Can you work these out from the model? Positions are in its coordinate system, mm. A direction names the side the tool comes from. Give positions to 0.01 mm unless a question says otherwise; leave off trailing zeros. Loops run counter-clockwise (first coordinate to the right, second up) from the corner with the lowest first, then second, coordinate; pieces in that order, holes last. Notation, with made-up numbers: M 20,7 L 45,7 A8 ccw 45,22 Z; hole C -23.5,70 d7. An arc over 180 degrees is marked long. Use CSV: the item, a comma, the result in double quotes.
from build123d import *

# Parameters (mm, degrees)
BOSS_EXTRUDE3_DEPTH  = 2.5
BOSS_EXTRUDE4_DEPTH  = 2.5
BOSS_EXTRUDE5_DEPTH  = 10.5
BOSS_EXTRUDE8_DEPTH  = 11
BOSS_EXTRUDE9_DEPTH  = 11
SKETCH8_W            = 84
SKETCH8_H            = 2
BOSS_EXTRUDE11_DEPTH = 4
SKETCH9_W            = 6
SKETCH9_H            = 7.053661792
CUT_EXTRUDE1_DEPTH   = 28
SKETCH10_W           = 6
SKETCH10_H           = 6.438726715
CUT_EXTRUDE4_DEPTH   = 11
SKETCH11_R           = 1.5
CUT_EXTRUDE5_DEPTH   = 14
SKETCH13_R           = 1.5
CUT_EXTRUDE6_DEPTH   = 14
SKETCH15_R           = 1.5
CUT_EXTRUDE7_DEPTH   = 14


with BuildPart() as part:
    # Sketch1 → Boss-Extrude3 (new body)
    with BuildSketch(Plane(origin=(0, 0, 0), x_dir=(1, 0, 0), z_dir=(0, 1, 0))):
        with BuildLine():
            Line((-44.72135955, -40), (0, -40))
            Line((0, -40), (44.72135955, -40))
            ThreePointArc((44.72135955, -40), (56.050341538, -21.409325386), (60, 0))
            ThreePointArc((60, 0), (-21.409325386, 56.050341538), (-44.72135955, -40))
        make_face()
        with BuildLine():
            Line((-33.166247904, -50), (0, -50))
            Line((0, -50), (0, -40))
            Line((0, -40), (-44.72135955, -40))
            ThreePointArc((-44.72135955, -40), (-39.2634671, -45.369374597), (-33.166247904, -50))
        make_face()
        with BuildLine():
            Line((0, -40), (0, -50))
            Line((0, -50), (33.166247904, -50))
            ThreePointArc((33.166247904, -50), (39.2634671, -45.369374597), (44.72135955, -40))
            Line((44.72135955, -40), (0, -40))
        make_face()
        with BuildLine():
            Line((0, -50), (0, -60))
            add(Edge.make_bspline(
                [(0, -60), (2.493909774, -59.986931125), (4.933150425, -59.785698627)],
                knots=[0, 0, 0, 0.138485859, 0.138485859, 0.138485859], degree=2))
            add(Edge.make_bspline(
                [(4.933150425, -59.785698627), (12.350363719, -59.151298506), (19.667130305, -57.122142348), (26.368544437, -53.878843782)],
                knots=[0.549095967, 0.549095967, 0.549095967, 0.549095967, 0.769976712, 0.769976712, 0.769976712, 0.769976712], degree=3))
            add(Edge.make_bspline(
                [(26.368544437, -53.878843782), (29.836187059, -52.176190697), (33.166247904, -50)],
                knots=[0.7803077, 0.7803077, 0.7803077, 1, 1, 1], degree=2))
            Line((33.166247904, -50), (0, -50))
        make_face()
        with BuildLine():
            add(Edge.make_bspline(
                [(-9.467287752, -59.24160526), (-4.836502075, -59.974590334), (0, -60)],
                knots=[0.731444001, 0.731444001, 0.731444001, 1, 1, 1], degree=2))
            Line((0, -60), (0, -50))
            Line((0, -50), (-33.166247904, -50))
            add(Edge.make_bspline(
                [(-33.166247904, -50), (-28.091057223, -53.316740978), (-22.696065652, -55.533505256)],
                knots=[0, 0, 0, 0.334842238, 0.334842238, 0.334842238], degree=2))
            add(Edge.make_bspline(
                [(-22.696065652, -55.533505256), (-18.44552317, -57.261077796), (-13.998129322, -58.510750178), (-9.467287752, -59.24160526)],
                knots=[0.269647974, 0.269647974, 0.269647974, 0.269647974, 0.406041898, 0.406041898, 0.406041898, 0.406041898], degree=3))
        make_face()
    extrude(amount=BOSS_EXTRUDE3_DEPTH)

    # Sketch3 → Boss-Extrude4 (add)
    with BuildSketch(Plane(origin=(0, 2.5, 0), x_dir=(1, 0, 0), z_dir=(0, 1, 0))):
        Polygon((0, 60), (-60, 60), (-60, -60), (60, -60), (60, 60), align=None)
    extrude(amount=-BOSS_EXTRUDE4_DEPTH)

    # Sketch4 → Boss-Extrude5 (add)
    with BuildSketch(Plane(origin=(0, 2.5, 0), x_dir=(1, 0, 0), z_dir=(0, 1, 0))):
        Polygon((3, 60), (0, 60), (-3, 60), (-3, -60), (3, -60), align=None)
    extrude(amount=BOSS_EXTRUDE5_DEPTH)

    # Sketch5 → Boss-Extrude8 (add)
    with BuildSketch(Plane(origin=(0, 2.5, 0), x_dir=(1, 0, 0), z_dir=(0, 1, 0))):
        Polygon((-43, -60), (-3, -60), (-3, -58), (-43, -58), (-43, 60), (-45, 60), (-45, -58), (-45, -60), align=None)
    extrude(amount=BOSS_EXTRUDE8_DEPTH)

    # Sketch7 → Boss-Extrude9 (add)
    with BuildSketch(Plane(origin=(0, 2.5, 0), x_dir=(1, 0, 0), z_dir=(0, 1, 0))):
        Polygon((3, -60), (43, -60), (43, 60), (41, 60), (41, -58), (3, -58), align=None)
    extrude(amount=BOSS_EXTRUDE9_DEPTH)

    # Sketch8 → Boss-Extrude11 (add)
    with BuildSketch(Plane(origin=(0, 2.5, 0), x_dir=(1, 0, 0), z_dir=(0, 1, 0))):
        with Locations((-1, 59)):
            Rectangle(SKETCH8_W, SKETCH8_H)
    extrude(amount=BOSS_EXTRUDE11_DEPTH)

    # Sketch9 → Cut-Extrude1 (cut)
    with BuildSketch(Plane(origin=(0, 2.5, 0), x_dir=(1, 0, 0), z_dir=(0, 1, 0))):
        with Locations((0, 56.473169104)):
            Rectangle(SKETCH9_W, SKETCH9_H)
    extrude(amount=CUT_EXTRUDE1_DEPTH, mode=Mode.SUBTRACT)

    # Sketch10 → Cut-Extrude4 (cut)
    with BuildSketch(Plane(origin=(0, 2.5, 0), x_dir=(1, 0, 0), z_dir=(0, 1, 0))):
        with Locations((0, 49.72697485)):
            Rectangle(SKETCH10_W, SKETCH10_H)
    extrude(amount=CUT_EXTRUDE4_DEPTH, mode=Mode.SUBTRACT)

    # Sketch11 → Cut-Extrude5 (cut)
    with BuildSketch(Plane(origin=(0, 2.5, 0), x_dir=(1, 0, 0), z_dir=(0, 1, 0))):
        with Locations(Location((-35.129064889, -35.129064889, 0), (0, 0, 270))):
            Circle(SKETCH11_R)
        with Locations(Location((35.129064889, -35.129064889, 0), (0, 0, 270))):
            Circle(SKETCH11_R)
    extrude(amount=-CUT_EXTRUDE5_DEPTH, mode=Mode.SUBTRACT)

    # Sketch13 → Cut-Extrude6 (cut)
    with BuildSketch(Plane(origin=(0, 13, 0), x_dir=(1, 0, 0), z_dir=(0, 1, 0))):
        with Locations(Location((-55, 0, 0), (0, 0, 270))):
            Circle(SKETCH13_R)
        with Locations(Location((55, 0, 0), (0, 0, 270))):
            Circle(SKETCH13_R)
    extrude(amount=-CUT_EXTRUDE6_DEPTH, mode=Mode.SUBTRACT)

    # Sketch15 → Cut-Extrude7 (cut)
    with BuildSketch(Plane(origin=(0, 2.5, 0), x_dir=(1, 0, 0), z_dir=(0, 1, 0))):
        with Locations(Location((0, 55, 0), (0, 0, 270))):
            Circle(SKETCH15_R)
    extrude(amount=-CUT_EXTRUDE7_DEPTH, mode=Mode.SUBTRACT)


solid = part.part
Q1. Please list where these lines run through material, in increasing order: L1, parallel to X at y = 11, z = 18; L2, parallel to X at y = 1.75, z = 0; L3, parallel to Z at x = 35.5, y = 4. Write a range as from..to.
Model answer:
L1,"-45..-43, -3..3, 41..43"
L2,"-60..-56.5, -53.5..53.5, 56.5..60"
L3,"-60..-58, 58..60"
Q2. I want a section at D-D, the plane z = -55. Please give me the cut outline in (x, y).
Model answer:
outline,"M -60,0 L -1.5,0 L -1.5,2.5 L -43,2.5 L -43,13.5 L -45,13.5 L -45,2.5 L -60,2.5 Z; M 1.5,0 L 60,0 L 60,2.5 L 43,2.5 L 43,13.5 L 41,13.5 L 41,2.5 L 1.5,2.5 Z"
Q3. For faces 1 (the flat face through (43, 8, 1)), 2 (the flat face through (0, 13, 6)), 3 (the flat face through (-43, 8, 0)), 4 (the flat face through (-53, 2.5, -1)), which set-ups out of +Z, -Z, +X, -X, +Y, -Y let a thin tool reach every point of the face, with its end or its side?
Model answer:
face 1,"+Z, -Z, +X, +Y"
face 2,"+Z, -Z, +Y"
face 3,"+Y"
face 4,"+Z, -Z, -X, +Y"
Q4. If we mould it in two halves opening along Z, with no side actions, what happens to faces 5 (the flat face through (-45, 8, -1)), 6 (the flat face through (-1, 7, 60)), 7 (the flat face through (22, 4, -58))? For each: released by +Z, released by -Z, zero draft, split by the parting line, or undercut.
Model answer:
face 5,"zero draft"
face 6,"released by +Z"
face 7,"undercut"
Q5. I want a section at A-A, the plane z = 0. Please give me the cut outline in (x, y).
Model answer:
outline,"M -60,0 L -56.5,0 L -56.5,2.5 L -60,2.5 Z; M -53.5,0 L 53.5,0 L 53.5,2.5 L 43,2.5 L 43,13.5 L 41,13.5 L 41,2.5 L 3,2.5 L 3,13 L -3,13 L -3,2.5 L -43,2.5 L -43,13.5 L -45,13.5 L -45,2.5 L -53.5,2.5 Z; M 56.5,0 L 60,0 L 60,2.5 L 56.5,2.5 Z"
Q6. I want a section at C-C, the plane y = 11. Please give me the cut outline in (x, z), then the cut area to 3 significant figures.
Model answer:
outline,"M -45,-60 L -43,-60 L -43,58 L -3,58 L -3,-46.51 L 3,-46.51 L 3,58 L 41,58 L 41,-60 L 43,-60 L 43,60 L -45,60 Z"
area,"1,280 mm2"
Q7. I want a section at B-B, the plane x = 0. Please give me the cut outline in (y, z), then the cut area to 3 significant figures.
Model answer:
outline,"M 0,-60 L 2.5,-60 L 2.5,-56.5 L 0,-56.5 Z; M 0,-53.5 L 2.5,-53.5 L 2.5,-46.51 L 13,-46.51 L 13,60 L 0,60 Z"
area,"1,410 mm2"
Q8. I'm going to push flat-ended pins straight in: P1, Ø5, axis at y = 9.5, z = -43.5, coming from the -X side; P2, Ø2, axis at x = -14.5, z = -59, coming from the +Y side; P3, Ø1, axis at y = 4.5, z = -59.5, coming from the +X side. Where does each tip first touch, or does it pass through?
Model answer:
P1,"x = -45"
P2,"y = 6.5"
P3,"x = 43"
